Geometry: final body of the model. Coordinates: model frame, mm. A direction names the side the tool comes from. Round coordinates to 2 decimals unless told otherwise and drop trailing zeros. Write each loop counter-clockwise with the first axis right and the second up, starting at its lowest first coordinate (ties: lowest second). Pieces come first, ordered by that corner, then holes. Notation, with made-up numbers: (-19.75, 32) - (9.25, 32) arc R11 cw to (9.25, 51) - close; hole circle Ø7 at (-18.5, 52). An arc over 180 degrees is marked (long way). Use a Markdown table: item, result. Add a question column.
```python
from build123d import *

# Parameters (mm, degrees)
F1_DEPTH = 51.054
F2_R     = 5.08


with BuildPart() as f1:
    # F0 (on Front) → F1 (new body)
    with BuildSketch(Plane.XZ):
        Polygon((-14.309117, 32.347076), (-64.300053, 32.347076), (-54.325373, -33.485826), (50.112445, -33.485826), (45.038836, 0), (-9.408046, 0), align=None)
    extrude(amount=F1_DEPTH)

    # F2
    f2_edges = [f1.edges().sort_by_distance(p)[0] for p in [
        (-39.304585, -51.054, 32.347076),
        (-59.312713, -51.054, -0.569375),
        (-2.106464, -51.054, -33.485826),
        (47.575641, -51.054, -16.742913),
        (17.815395, -51.054, 0),
        (-11.858581, -51.054, 16.173538),
        (-39.304585, 0, 32.347076),
        (-59.312713, 0, -0.569375),
        (-2.106464, 0, -33.485826),
        (47.575641, 0, -16.742913),
        (17.815395, 0, 0),
        (-11.858581, 0, 16.173538),
        (-9.408046, -25.527, 0),
        (-14.309117, -25.527, 32.347076),
        (45.038836, -25.527, 0),
        (50.112445, -25.527, -33.485826),
        (-64.300053, -25.527, 32.347076),
    ]]
    fillet(f2_edges, radius=F2_R)


solid = f1.part
```
1) Draft query along X for faces 1 (the cylindrical face through (48.02, -25.81, -31.76)), 2 (the cylindrical face through (17.495, -1.528, -1.449)), 3 (the flat face through (-58.934, -25.241, -3.07)). Return one class per face: released by +X, released by -X, zero draft, split by the parting line, or undercut.
2) Section B-B, the plane y = -20. Return the cut outline in (x, z).
3) Pin query (flat end, axial travel): P1, Ø10, axis at y = -27, z = -11, coming from the -X side; P2, Ø10, axis at y = -45, z = -20.5, coming from the +X side; P3, Ø20.5, axis at x = 28, y = -20, coming from the +Z side. Return the tip coordinate at first contact, or that it passes through.
4) Section A-A, the plane x = 12.5. Return the cut outline in (y, z), then the cut area to 3 significant figures.
5) Set-up query: faces 4 (the flat face through (18, -25, 0)), 5 (the flat face through (-6, -25, -33.486)). Return all of +Z, -Z, +X, -X, +Y, -Y with unobstructed straight access to the full face (end or side cutting, diameter ignored); none if empty.
6) Material intervals for L1, parallel to Z at x = 32.5, y = -26.5; L2, parallel to Y at x = -55.5, z = -1; L3, parallel to X at y = -44, z = -1.5, sorted ascending. Write a range as from..to.
Output values:
| question | item | result |
|---|---|---|
| 1 | face 1 | released by +X |
| 1 | face 2 | zero draft |
| 1 | face 3 | released by -X |
| 2 | outline | (-63.42, 26.51) - (-54.33, -33.49) - (44.2, -33.49) arc R5.08 ccw to (49.23, -27.64) - (45.69, -4.32) arc R5.08 ccw to (40.67, 0) - (-5.04, 0) arc R5.08 cw to (-10.06, 4.32) - (-13.65, 28.03) arc R5.08 ccw to (-18.68, 32.35) - (-58.39, 32.35) arc R5.08 ccw to start |
| 3 | P1 | stops at x = -58.49 |
| 3 | P2 | stops at x = 48.9 |
| 3 | P3 | stops at z = 0 |
| 4 | outline | (-51.05, -28.41) arc R5.08 ccw to (-45.97, -33.49) - (-5.08, -33.49) arc R5.08 ccw to (0, -28.41) - (0, -5.08) arc R5.08 ccw to (-5.08, 0) - (-45.97, 0) arc R5.08 ccw to (-51.05, -5.08) - close |
| 4 | area | 1,690 mm^2 |
| 5 | face 4 | +Z, +X, +Y, -Y |
| 5 | face 5 | -Z, +X, -X, +Y, -Y |
| 6 | L1 | z = -33.49..0 |
| 6 | L2 | y = -50.86..-0.19 |
| 6 | L3 | x = -59.17..44.27 |
